Part print with two shaded views. Sizes in mm from the minimum x, y, z corner. Round coordinates to 2 decimals unless told otherwise and drop trailing zeros. Loops run counter-clockwise (first coordinate to the right, second up) from the corner with the lowest first, then second, coordinate; pieces in that order, holes last.
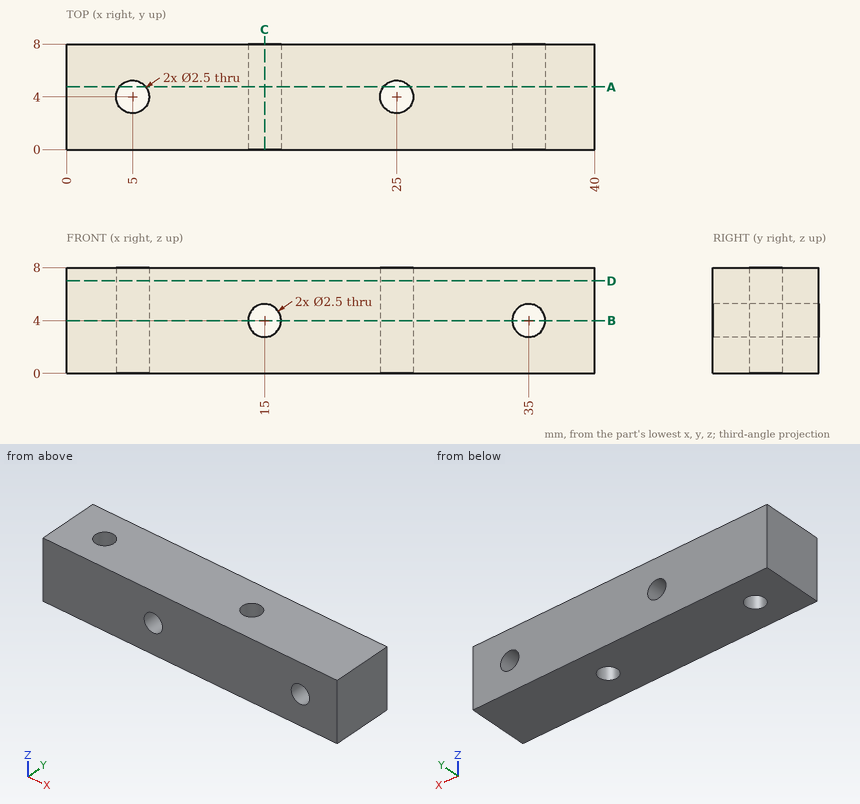
Item 1: Cut at C-C (x = 15). List the corners of the cut face in (y, z).
Verdict:
outline: (0, 0) - (8, 0) - (8, 2.75) - (0, 2.75) - close; (0, 5.25) - (8, 5.25) - (8, 8) - (0, 8) - close
Item 2: Cut at D-D (z = 7). List the corners of the cut face in (x, y), plus the area to 3 significant figures.
Verdict:
outline: (0, 0) - (40, 0) - (40, 8) - (0, 8) - close; hole circle Ø2.5 at (5, 4); hole circle Ø2.5 at (25, 4)
area: 310 mm2
Item 3: Flat gauge pins, fed straight in: P1, Ø3, axis at x = 29.5, y = 2.5, coming from the -Z side; P2, Ø2, axis at x = 15, z = 4, coming from the +Y side. Where does each tip first touch, or does it go through?
Verdict:
P1: stops at z = 0
P2: passes through
Item 4: Cut at B-B (z = 4). List the corners of the cut face in (x, y), plus the area to 3 significant figures.
Verdict:
outline: (0, 0) - (13.75, 0) - (13.75, 8) - (0, 8) - close; (16.25, 0) - (33.75, 0) - (33.75, 8) - (16.25, 8) - close; (36.25, 0) - (40, 0) - (40, 8) - (36.25, 8) - close; hole circle Ø2.5 at (5, 4); hole circle Ø2.5 at (25, 4)
area: 270 mm2
Item 5: Cut at A-A (y = 4.75). List the corners of the cut face in (x, z), plus the area to 3 significant figures.
Verdict:
outline: (0, 0) - (4, 0) - (4, 8) - (0, 8) - close; (6, 0) - (24, 0) - (24, 8) - (6, 8) - close; (26, 0) - (40, 0) - (40, 8) - (26, 8) - close; hole circle Ø2.5 at (15, 4); hole circle Ø2.5 at (35, 4)
area: 278 mm2
Item 6: Wall check: L1, parallel to X at y = 3.75, z = 2; L2, parallel to Y at x = 5, z = 5.5; L3, parallel to X at y = 3, z = 4. Give the ranges that are in metal, low to high.
Verdict:
L1: x = 0 to 3.78, 6.22 to 23.78, 26.22 to 40
L2: y = 0 to 2.75, 5.25 to 8
L3: x = 0 to 4.25, 5.75 to 13.75, 16.25 to 24.25, 25.75 to 33.75, 36.25 to 40
